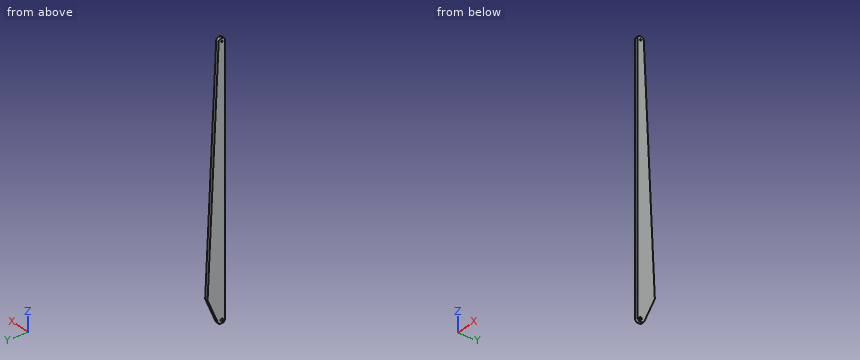
from build123d import *

# Parameters (mm, degrees)
SKETCH3_R           = 1.6002
SKETCH3_R_2         = 2.5527
BOSS_EXTRUDE1_DEPTH = 6.35
FILLET1_R           = 5.08


with BuildPart() as part:
    # Sketch3 → Boss-Extrude1 (new body)
    with BuildSketch(Plane(origin=(0, 0, 0), x_dir=(0, 0, -1), z_dir=(1, 0, 0))):
        Polygon((-265.049, 0), (265.049, 0), (277.749, 0), (277.749, 12.7), (221.687563823, 36.153126397), (-277.749, 12.7), (-277.749, 0), align=None)
        with Locations((-271.399, 6.35)):
            Circle(SKETCH3_R, mode=Mode.SUBTRACT)
        with Locations((271.399, 6.35)):
            Circle(SKETCH3_R_2, mode=Mode.SUBTRACT)
    extrude(amount=BOSS_EXTRUDE1_DEPTH)

    # Fillet1
    fillet1_edges = [part.edges().sort_by_distance(p)[0] for p in [
        (3.175, 0, 277.749),
        (3.175, 12.7, 277.749),
        (3.175, 36.153126397, -221.687563823),
        (3.175, 12.7, -277.749),
        (3.175, 0, -277.749),
    ]]
    fillet(fillet1_edges, radius=FILLET1_R)


solid = part.part
Read the model definition and answer for the solid it produces. Units are mm, in the model's axes. Give positions to 0.01 mm unless a question says otherwise; leave off trailing zeros. Write each loop counter-clockwise with the first axis right and the second up, starting at its lowest first coordinate (ties: lowest second). Pieces come first, ordered by that corner, then holes. Notation, with made-up numbers: (87.5, 36.25) - (143.5, 36.25) arc R22 cw to (143.5, 56.25) - close; hole circle Ø5 at (22, 63). An arc over 180 degrees is marked (long way). Return JSON: item names as keys, results as strings.
Q1. A cutting plane is placed at C-C, the plane y = 19. Determine the outline of the cut face in (x, z).
Reply:
{"outline": "(0, -262.69) - (6.35, -262.69) - (6.35, 143.59) - (0, 143.59) - close"}
Q2. A cutting plane is placed at B-B, the plane z = 94.5. Determine the outline of the cut face in (x, y).
Reply:
{"outline": "(0, 0) - (6.35, 0) - (6.35, 21.31) - (0, 21.31) - close"}
Q3. Given P1, Ø3, axis at x = 2.5, z = -121.5, coming from the +Y side; P2, Ø8, axis at y = 6.35, z = -271.399, coming from the -X side; P3, Ø2, axis at x = 2, z = 118, coming from the +Y side; P4, Ø1.5, axis at x = 3.5, z = 79.5, coming from the +Y side, each flat-ended and moving along its own axis, determine where each tip first touches the part or whether it passes through.
Reply:
{"P1": "y = 31.52", "P2": "x = 0", "P3": "y = 20.25", "P4": "y = 22.04"}
Q4. Consider line 1 along Z through (x, y) = (1.75, 4); line 2 along Z through (x, y) = (4, 8); line 3 along Y through (x, z) = (2, 146). Determine where each line is inside the solid, lowest interval first. Write a range as [from, to].
Reply:
{"line 1": "[-277.63, -272.4], [-270.4, 277.63]", "line 2": "[-277.75, -273.35], [-269.45, 277.75]", "line 3": "[0, 18.89]"}
Q5. A cutting plane is placed at A-A, the plane x = 5. Determine the outline of the cut face in (y, z).
Reply:
{"outline": "(0, -272.67) arc R5.08 ccw to (5.08, -277.75) - (9.32, -277.75) arc R5.08 ccw to (14.01, -274.63) - (35.71, -222.74) arc R5.08 ccw to (36.1, -220.54) - (12.93, 272.91) arc R5.08 ccw to (7.85, 277.75) - (5.08, 277.75) arc R5.08 ccw to (0, 272.67) - close; hole circle Ø5.11 at (6.35, -271.4); hole circle Ø3.2 at (6.35, 271.4)"}
